Here's the drawing with two shaded views (mm, measured from the low corner). I have some questions. Give positions to 0.01 mm unless a question says otherwise; leave off trailing zeros. Write each loop counter-clockwise with the first axis right and the second up, starting at its lowest first coordinate (ties: lowest second). Pieces come first, ordered by that corner, then holes. Notation, with made-up numbers: (88, 10) - (94, 10) arc R20 cw to (94, 44) - close; hole circle Ø9 at (0, 33.5). An arc over 180 degrees is marked (long way). Answer as CSV lines item,"result". Start each with the question number.
Q1. Imagine slicing it at A-A on z = 15.5. List the corners of the cut face in (x, y) for me (1 decimal).
Q2. Imagine slicing it at B-B on y = 2.45. State how many separate pieces and enclosed holes the cut face has, and give its area (3 significant figures).
Q3. If I drill on line 1 along X through (y, z) = (2.75, 23.5); line 2 along X through (y, z) = (2.45, 14); line 3 along X through (y, z) = (1.5, 32), over which ranges is the centre line in solid material (lowest first)?
Q4. Imagine slicing it at C-C on z = 7.5. List the corners of the cut face in (x, y) for me (1 decimal).
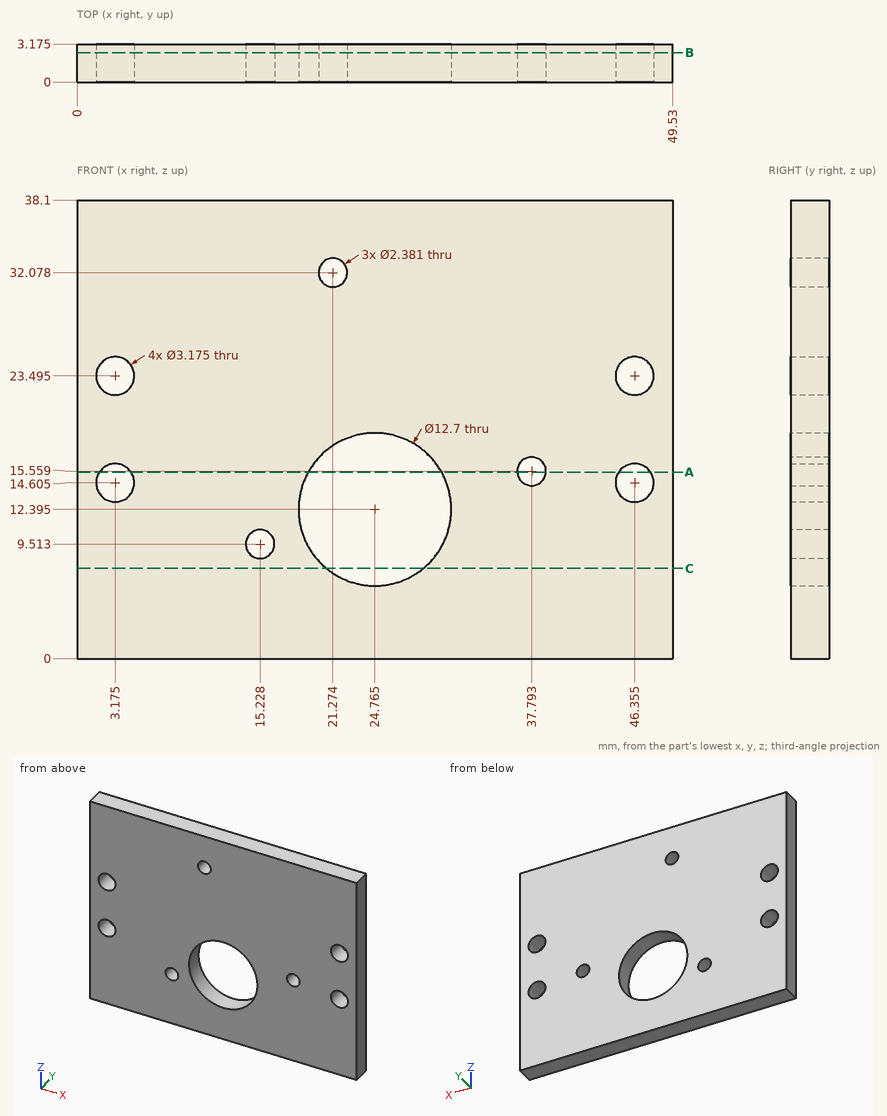
Conclusion:
1,outline,"(0, 0) - (1.9, 0) - (1.9, 3.2) - (0, 3.2) - close; (4.5, 0) - (19.2, 0) - (19.2, 3.2) - (4.5, 3.2) - close; (30.3, 0) - (36.6, 0) - (36.6, 3.2) - (30.3, 3.2) - close; (39, 0) - (45, 0) - (45, 3.2) - (39, 3.2) - close; (47.7, 0) - (49.5, 0) - (49.5, 3.2) - (47.7, 3.2) - close"
2,separate pieces,"1"
2,enclosed holes,"8"
2,area,"1,720 mm^2"
3,line 1,"0 to 1.59, 4.76 to 44.77, 47.94 to 49.53"
3,line 2,"0 to 1.71, 4.64 to 18.62, 30.91 to 44.89, 47.82 to 49.53"
3,line 3,"0 to 20.09, 22.46 to 49.53"
4,outline,"(0, 0) - (20.7, 0) - (20.7, 3.2) - (0, 3.2) - close; (28.8, 0) - (49.5, 0) - (49.5, 3.2) - (28.8, 3.2) - close"
